Here's how the part is built. I have some questions about the finished solid (model axes, mm). A direction names the side the tool comes from. Round coordinates to 2 decimals unless told otherwise and drop trailing zeros. Write each loop counter-clockwise with the first axis right and the second up, starting at its lowest first coordinate (ties: lowest second). Pieces come first, ordered by that corner, then holes. Notation, with made-up numbers: (35, 70.25) -> (74, 70.25) arc R18 ccw to (74, 97.25) -> close; hole circle Ø8 at (63, 18). An arc over 180 degrees is marked (long way). Answer in a Markdown table with one row per item.
from build123d import *

# Parameters (mm, degrees)
F0_W      = 40
F0_H      = 72
F1_DEPTH  = 36
F2_W      = 5.110045895
F2_H      = 2.0075347275
F2_W_2    = 5.1063122059
F2_W_3    = 5.1025785169
F2_W_4    = 5.0988448278
F2_W_5    = 5.0951111388
F2_W_6    = 5.0913774498
F2_W_7    = 5.0876437607
F2_W_8    = 5.0839100717
F2_W_9    = 5.0801763826
F2_W_10   = 5.0764426936
F2_W_11   = 5.0727090045
F2_W_12   = 5.0689753155
F2_W_13   = 1.42415151
F2_H_2    = 3.0305987895
F2_R      = 10.5
F2_R_2    = 10
F3_DEPTH  = 10
F4_W      = 7.6698157936
F4_H      = 0.7368782535
F5_DEPTH  = 2
F6_W      = 21.4133905619
F6_H      = 21.0468042642
F7_DEPTH  = 15
F9_DEPTH  = 50
F10_R     = 2.4823069634
F11_DEPTH = 5
F12_R     = 2


with BuildPart() as f1:
    # F0 (on Front) → F1 (new body)
    with BuildSketch(Plane.XZ):
        with Locations((-13.0052822828, -9.5213338137)):
            Rectangle(F0_W, F0_H)
    extrude(amount=F1_DEPTH)

    # F2 (on face) → F3 (cut)
    with BuildSketch(Plane.XZ.offset(36)):
        with Locations((-30.4502593353, 22.1199980006)):
            Rectangle(F2_W, F2_H)
        with Locations((-30.4521261799, 18.6199999921)):
            Rectangle(F2_W_2, F2_H)
        with Locations((-30.4539930244, 15.1200019835)):
            Rectangle(F2_W_3, F2_H)
        with Locations((-30.4558598689, 11.620003975)):
            Rectangle(F2_W_4, F2_H)
        with Locations((-30.4577267134, 8.1200059665)):
            Rectangle(F2_W_5, F2_H)
        with Locations((-30.459593558, 4.620007958)):
            Rectangle(F2_W_6, F2_H)
        with Locations((-30.4614604025, 1.1200099495)):
            Rectangle(F2_W_7, F2_H)
        with Locations((-30.463327247, -2.379988059)):
            Rectangle(F2_W_8, F2_H)
        with Locations((-30.4651940915, -5.8799860675)):
            Rectangle(F2_W_9, F2_H)
        with Locations((-30.467060936, -9.379984076)):
            Rectangle(F2_W_10, F2_H)
        with Locations((-30.4689277806, -12.8799820845)):
            Rectangle(F2_W_11, F2_H)
        with Locations((-30.4707946251, -16.379980093)):
            Rectangle(F2_W_12, F2_H)
        with Locations((4.4602300594, -16.379980093)):
            Rectangle(F2_W_12, F2_H)
        with Locations((4.4583632149, -12.8799820845)):
            Rectangle(F2_W_11, F2_H)
        with Locations((4.4564963704, -9.379984076)):
            Rectangle(F2_W_10, F2_H)
        with Locations((4.4546295259, -5.8799860675)):
            Rectangle(F2_W_9, F2_H)
        with Locations((4.4508958368, 1.1200099495)):
            Rectangle(F2_W_7, F2_H)
        with Locations((4.4490289923, 4.620007958)):
            Rectangle(F2_W_6, F2_H)
        with Locations((4.4471621478, 8.1200059665)):
            Rectangle(F2_W_5, F2_H)
        with Locations((4.4452953032, 11.620003975)):
            Rectangle(F2_W_4, F2_H)
        with Locations((4.4434284587, 15.1200019835)):
            Rectangle(F2_W_3, F2_H)
        with Locations((4.4415616142, 18.6199999921)):
            Rectangle(F2_W_2, F2_H)
        with Locations((4.4396947697, 22.1199980006)):
            Rectangle(F2_W, F2_H)
        with Locations((0.9947177172, 24.9633667916)):
            Rectangle(F2_W_13, F2_H_2)
        with Locations((-2.5052822828, 24.9633667916)):
            Rectangle(F2_W_13, F2_H_2)
        with Locations((-6.0052822828, 24.9633667916)):
            Rectangle(F2_W_13, F2_H_2)
        with Locations((-9.5052822828, 24.9633667916)):
            Rectangle(F2_W_13, F2_H_2)
        with Locations((-16.5052822828, 24.9633667916)):
            Rectangle(F2_W_13, F2_H_2)
        with Locations((-20.0052822828, 24.9633667916)):
            Rectangle(F2_W_13, F2_H_2)
        with Locations((-23.5052822828, 24.9633667916)):
            Rectangle(F2_W_13, F2_H_2)
        with Locations((-27.0052822828, 24.9633667916)):
            Rectangle(F2_W_13, F2_H_2)
        with Locations((4.4527626813, -2.379988059)):
            Rectangle(F2_W_8, F2_H)
        with Locations((-13.0316922441, 6.5578259528)):
            Circle(F2_R)
        with Locations((-13.0316922441, 6.5578259528)):
            Circle(F2_R_2, mode=Mode.SUBTRACT)
    extrude(amount=-F3_DEPTH, mode=Mode.SUBTRACT)

    # F4 (on face) → F5 (cut)
    with BuildSketch(Plane.XZ.offset(36)):
        with Locations((-13.0316922441, 6.5578259528)):
            Rectangle(F4_W, F4_H)
    extrude(amount=-F5_DEPTH, mode=Mode.SUBTRACT)

    # F6 (on face) → F7 (cut)
    with BuildSketch(Plane.XZ.offset(36)):
        with Locations((-13.0052822828, -34.9979316816)):
            Rectangle(F6_W, F6_H)
    extrude(amount=-F7_DEPTH, mode=Mode.SUBTRACT)

    # F8 (on face) → F9 (cut)
    with BuildSketch(Plane.YZ.offset(6.9947177172)):
        Polygon((-29.6883769333, -45.5213338137), (-36, -23.9366423339), (-36, -45.5213338137), align=None)
    extrude(amount=-F9_DEPTH, mode=Mode.SUBTRACT)

    # F10 (on face) → F11 (cut)
    with BuildSketch(Plane.XZ.offset(36)):
        with Locations((-18.7515150756, -15.9784462303)):
            Circle(F10_R)
        with Locations((-7.2590494901, -15.9784462303)):
            Circle(F10_R)
    extrude(amount=-F11_DEPTH, mode=Mode.SUBTRACT)

    # F12
    f12_edges = [f1.edges().sort_by_distance(p)[0] for p in [
        (-33.005282, -36, 24.801216),
        (-33.005282, -36, 20.369999),
        (-33.005282, -36, 16.870001),
        (-33.005282, -36, 13.370003),
        (-33.005282, -36, 9.870005),
        (-33.005282, -36, 6.370007),
        (-33.005282, -36, 2.870009),
        (-33.005282, -36, -0.629989),
        (-33.005282, -36, -4.129987),
        (-33.005282, -36, -7.629985),
        (-33.005282, -36, -11.129983),
        (-33.005282, -36, -14.629981),
        (-33.005282, -36, -20.660195),
        (-33.005282, -32.844188, -34.728988),
        (6.994718, -36, 24.801216),
        (6.994718, -36, 20.369999),
        (6.994718, -36, 16.870001),
        (6.994718, -36, 13.370003),
        (6.994718, -36, 9.870005),
        (6.994718, -36, 6.370007),
        (6.994718, -36, 2.870009),
        (6.994718, -36, -0.629989),
        (6.994718, -36, -4.129987),
        (6.994718, -36, -7.629985),
        (6.994718, -36, -11.129983),
        (6.994718, -36, -14.629981),
        (6.994718, -36, -20.660195),
        (6.994718, -32.844188, -34.728988),
    ]]
    fillet(f12_edges, radius=F12_R)


solid = f1.part
1) I need wall thicknesses on line 1 (Z direction, x = -9, y = -34); line 2 (X direction, y = -27, z = 4); line 3 (X direction, y = -27, z = 2). Which ranges of each line are inside material? Lowest first, please. Write a range as [from, to].
Response:
| item | result |
|---|---|
| line 1 | z = [-24.47, -17.75], [-14.21, -3.14], [-2.59, 15.71], [16.25, 23.45] |
| line 2 | x = [-27.91, -23.22], [-22.7, -3.36], [-2.85, 1.9] |
| line 3 | x = [-27.92, -22.49], [-21.93, -4.13], [-3.57, 1.91] |
2) For pin 1 (5.5 mm diameter, centred on x = -31, y = -32, fed in from -Z); pin 2 (5 mm diameter, centred on x = -19, y = -28, fed in from -Z); pin 3 (1 mm diameter, centred on y = -32, z = 8.5, fed in from +X); pin 4 (0.6 mm diameter, centred on x = -30, z = 15.5, fed in from -Y), each with a flat end and sliding along its axis, tell me the tip position at first contact or that it passes through.
Response:
| item | result |
|---|---|
| pin 1 | stops at z = -45.52 |
| pin 2 | stops at z = -24.47 |
| pin 3 | stops at x = 1.9 |
| pin 4 | stops at y = -26 |
3) Which directions (+Z, -Z, +X, -X, +Y, -Y) give clear straight access to the entire face, cutting with the end or side of a thin tool? Please do faces 1 (the face through (-30, -31, 5.624)), 2 (the face through (-0.75, -32.8, -34.88)), 3 (the face through (-24, -31, 23.448)), 4 (the face through (4, -31, 12.624)).
Response:
| item | result |
|---|---|
| face 1 | -X, -Y |
| face 2 | -Z, +X, -X, -Y |
| face 3 | +Z, -Y |
| face 4 | +X, -Y |
4) We'd pull the mould along X, two halves only. Please class faces 5 (the face through (-27.925, -31, -6)), 6 (the face through (-7, -31, -16)), 7 (the face through (-31, -31, -4.876)): +X half, -X half, draft (parallel to the pull), parting line (faces both ways), or undercut.
Response:
| item | result |
|---|---|
| face 5 | -X half |
| face 6 | undercut |
| face 7 | draft |
5) I want a section at A-A, the plane y = -25. List the corners of the cut face in (x, z) for me.
Response:
| item | result |
|---|---|
| outline | (-33.01, -45.52) -> (-23.71, -45.52) -> (-23.71, -24.47) -> (-2.3, -24.47) -> (-2.3, -45.52) -> (6.99, -45.52) -> (6.99, 26.48) -> (-33.01, 26.48) -> close |
